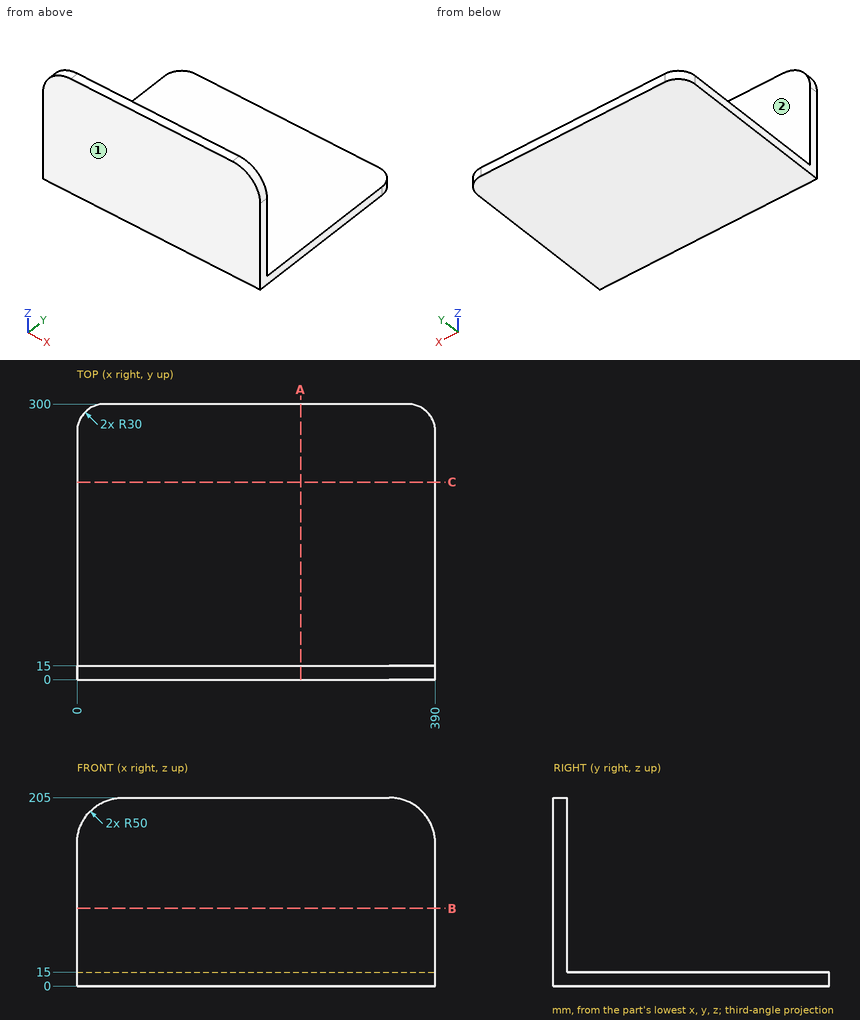
Part print with two shaded views. Sizes in mm from the minimum x, y, z corner. A direction names the side the tool comes from. Coordinates: 2 decimals unless noted, no trailing zeros. Order: outer loops, then holes, each group sorted by start corner. A loop starts at its lowest first (then second) coordinate and runs counter-clockwise, first axis right, second up. Notation, with made-up numbers: M 74,-38 L 104,-38 A22 ccw 104,-19 Z; hole C 16.5,74.5 d6. An arc over 180 degrees is marked long. One line per question, with ' | ' between items. Start each with the question number.
1. Flat gauge pins, fed straight in: P1, Ø1.5, axis at x = 100.5, y = 71.5, coming from the +Z side; P2, Ø2, axis at x = 159.5, z = 128.5, coming from the +Y side. Where does each tip first touch, or does it go through?
2. Cut at B-B (z = 84.5). Write the cut outline in (x, y), plus the area to 3 significant figures.
3. Tool access for the marked faces 1 and 2: list every direction of +Z, -Z, +X, -X, +Y, -Y with a clear straight run to the whole face (end or side of a thin tool).
4. Cut at A-A (x = 243.5). Write the cut outline in (y, z), plus the area to 3 significant figures.
5. Wall check: line 1 along Y through (x, z) = (128, 108). Give the ranges that are in metal, low to high. Write a range as [from, to].
The answers:
1) P1: stops at z = 15 | P2: stops at y = 15
2) outline: M 0,0 L 390,0 L 390,15 L 0,15 Z | area: 5,850 mm2
3) face 1: +Z, -Z, +X, -X, -Y | face 2: +Z, +X, -X, +Y
4) outline: M 0,0 L 300,0 L 300,15 L 15,15 L 15,205 L 0,205 Z | area: 7,350 mm2
5) line 1: y = [0, 15]
